Read the model definition and answer for the solid it produces. Units are mm, in the model's axes. Face numbers are marked on the shaded views. A direction names the side the tool comes from. Give positions to 0.01 mm unless a question says otherwise; leave off trailing zeros. Loops run counter-clockwise (first coordinate to the right, second up) from the corner with the lowest first, then second, coordinate; pieces in that order, holes last. Notation, with made-up numbers: (-31, 68) -> (-15, 68) arc R11 cw to (-15, 82) -> close; hole circle Ø4 at (5, -20.75). An arc over 180 degrees is marked (long way). Answer as CSV lines item,"result". Start each with the question number.
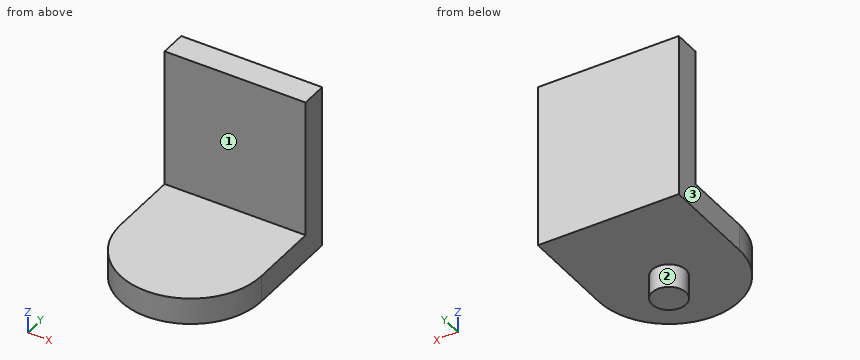
```python
from build123d import *

# Parameters (mm, degrees)
F1_DEPTH = 9.525
F0_W     = 50.8
F0_H     = 9.525
F2_DEPTH = 59.2582
F3_R     = 6.096
F4_DEPTH = 8.4582


with BuildPart() as f1:
    # F0 (on Top) → F1 (new body)
    with BuildSketch(Plane.XY):
        with BuildLine():
            Line((25.4, 25.4), (-25.4, 25.4))
            Line((-25.4, 25.4), (-25.4, 0))
            ThreePointArc((-25.4, 0), (0, -25.4), (25.4, 0))
            Line((25.4, 0), (25.4, 25.4))
        make_face()
    extrude(amount=F1_DEPTH)

    # F0 (on Top) → F2 (join)
    with BuildSketch(Plane.XY):
        with Locations((0, 30.1625)):
            Rectangle(F0_W, F0_H)
    extrude(amount=F2_DEPTH)

    # F3 (on face) → F4 (join)
    with BuildSketch(Plane.XY):
        Circle(F3_R)
    extrude(amount=-F4_DEPTH)


solid = f1.part
```
(1) A tool of negligible diameter and unlimited length cuts with its end or side. For the marked faces 1, 2 and 3, from which of +Z, -Z, +X, -X, +Y, -Y can it reach the whole face along a straight path? Write none if from no direction.
(2) Each of these flat-tipped pins is pushed along its axis until it touches: P1, Ø5, axis at x = 15.5, y = -16.5, coming from the -Z side; P2, Ø5, axis at x = -17, y = 19.5, coming from the +Z side (3 decimals); P3, Ø1.5, axis at x = -5, z = 35, coming from the -Y side. Where does it stop, or does it pass through?
(3) Find the intervals of material crossed by line 1 along Y through (x, z) = (-14.5, 42) (3 decimals); line 2 along Z through (x, y) = (-8.5, 30); line 3 along Z through (x, y) = (12.5, -3.5) (3 decimals), in increasing order. Write a range as from..to.
(4) Find section B-B on z = -3. Write down the section's boundary in (x, y), then the cut area to 3 significant figures.
(5) Find section D-D on x = -15. Write down the section's boundary in (y, z) (3 decimals), then the cut area to 3 significant figures.
(6) Find section A-A on x = 0. Write down the section's boundary in (y, z) (3 decimals).
(7) Find section C-C on y = 19. Write down the section's boundary in (x, z) (3 decimals).
Answer block:
1,face 1,"+Z, +X, -X, -Y"
1,face 2,"-Z"
1,face 3,"+Z, -Z, -X, +Y, -Y"
2,P1,"stops at z = 0"
2,P2,"stops at z = 9.525"
2,P3,"stops at y = 25.4"
3,line 1,"y = 25.4..34.925"
3,line 2,"z = 0..59.26"
3,line 3,"z = 0..9.525"
4,outline,"circle Ø12.19 at (0, 0)"
4,area,"117 mm2"
5,outline,"(-20.498, 0) -> (34.925, 0) -> (34.925, 59.258) -> (25.4, 59.258) -> (25.4, 9.525) -> (-20.498, 9.525) -> close"
5,area,"1,000 mm2"
6,outline,"(-25.4, 0) -> (-6.096, 0) -> (-6.096, -8.458) -> (6.096, -8.458) -> (6.096, 0) -> (34.925, 0) -> (34.925, 59.258) -> (25.4, 59.258) -> (25.4, 9.525) -> (-25.4, 9.525) -> close"
7,outline,"(-25.4, 0) -> (25.4, 0) -> (25.4, 9.525) -> (-25.4, 9.525) -> close"
